Read the model definition and answer for the solid it produces. Units are mm, in the model's axes. A direction names the side the tool comes from. Coordinates: 2 decimals unless noted, no trailing zeros. Write each loop counter-clockwise with the first axis right and the second up, starting at its lowest first coordinate (ties: lowest second). Pieces come first, ordered by that corner, then holes.
(1) Which of the six approach directions +Z, -Z, +X, -X, +Y, -Y give full straight-line access (tool end or side, diameter ignored) to faces 1 (the flat face through (-7, 7, -49)), 2 (the flat face through (-13, 7, -49)), 3 (the flat face through (16, -15, 37.5)), 4 (the flat face through (0, -18, 20)), 5 (the flat face through (-6, 15, -27.5))?
(2) The mould has two halves that part along Z. Classify faces 6 (the cylindrical face through (-35.994, 14.93, -57.236)), 7 (the flat face through (11, 10, 57)), 8 (the flat face through (-16, -16, -3)): +Z half, -Z half, draft (parallel to the pull), parting line (faces both ways), or undercut.
(3) Section A-A on x = 20 is taken. Write down the section's boundary in (y, z), then the cut area to 4 significant figures.
(4) Section C-C on z = -57.5 is taken. Write down the section's boundary in (x, y).
(5) Find the intervals of material crossed by probe 1 along Z at (x, y) = (20, 17); probe 2 along Z at (x, y) = (35, 13); probe 3 along Y at (x, z) = (20, 11), in increasing order.
(6) Section B-B on y = 15 is taken. Write down the section's boundary in (x, z), then the cut area to 3 significant figures.
(7) Section D-D on x = -30 is taken. Write down the section's boundary in (y, z).
(8) Given pin 1 (3 mm diameter, centred on y = 7, z = 57, fed in from +X); pin 2 (3 mm diameter, centred on y = -40, z = -15, fed in from +X); pin 3 (14 mm diameter, centred on x = 20, z = -57.5, fed in from -Y), each flat-ended and moving along its own axis, determine where each tip first touches the part or whether it passes through.
Solid Edge part; units mm, degrees
sketch "Sketch1" plane through (0, 0, 0) normal (0, 0, 1) x (1, 0, 0)
  line L0 (-50, 0) -> (0, 0)
  line L1 (0, 0) -> (0, -36.6)
  arc A0 (0, -36.6) -> (40, -36.6) centre (20, -36.6) ccw
  line L2 (-50, 0) -> (6.5476, -51.3997)
extrude "Protrusion1" add sketch "Sketch1" along normal mid plane 6 material side at (-25, -0.05, 0)
sketch "Sketch2" plane through (0, 0, 0) normal (0, 0, 1) x (1, 0, 0)
  line L0 (40, 20) -> (-50, 20)
  line L1 (-50, 20) -> (-50, 0)
  line L2 (-50, 0) -> (0, 0)
  line L3 (0, 0) -> (0, -36.6)
  arc A0 (0, -36.6) -> (40, -36.6) centre (20, -36.6) ccw
  line L4 (40, -36.6) -> (40, 20)
  circle A1 centre (20, -36.6) radius 10
extrude "ExtrudedProtrusion_2" add sketch "Sketch2" along normal mid plane 75
sketch "Sketch3" plane through (0, 0, 0) normal (0, 0, 1) x (1, 0, 0)
  line L0 (-50, 10) -> (40, 10)
  line L1 (40, 10) -> (40, 20)
  line L2 (40, 20) -> (-50, 20)
  line L3 (-50, 20) -> (-50, 10)
extrude "ExtrudedCutout_4" cut sketch "Sketch3" along normal mid plane 55
sketch "Sketch4" plane through (-5, -18.3, 37.5) normal (0, 0, 1) x (0, 1, 0)
  line L0 (38.3, 45) -> (28.3, 45)
  line L1 (28.3, 45) -> (28.3, -45)
  line L2 (28.3, -45) -> (38.3, -45)
  line L3 (38.3, -45) -> (38.3, 45)
extrude "ExtrudedProtrusion_5" add sketch "Sketch4" along normal blind 40
sketch "Sketch5" plane through (40, 20, -37.5) normal (0, 0, -1) x (0, -1, 0)
  line L0 (10, 0) -> (0, 0)
  line L1 (0, 0) -> (0, 90)
  line L2 (0, 90) -> (10, 90)
  line L3 (10, 90) -> (10, 0)
extrude "ExtrudedProtrusion_6" add sketch "Sketch5" along normal blind 40
sketch "Sketch6" plane through (-5, 10, 57.5) normal (0, -1, 0) x (1, 0, 0)
  circle A0 centre (25, 0) radius 6
  circle A1 centre (-25, 0) radius 6
  circle A2 centre (25, -115) radius 6
  circle A3 centre (-25, -115) radius 6
extrude "ExtrudedCutout_5" cut sketch "Sketch6" against normal blind 100
sketch "Sketch7" plane through (-13, 10, 0) normal (-1, 0, 0) x (0, 0, -1)
  line L0 (-77.5, 0) -> (-37.5, 10)
  line L1 (-37.5, 10) -> (-37.5, 0)
  line L2 (-37.5, 0) -> (-77.5, 0)
  line L3 (37.5, 10) -> (77.5, 0)
  line L4 (77.5, 0) -> (37.5, 0)
  line L5 (37.5, 0) -> (37.5, 10)
extrude "ExtrudedProtrusion_7" add sketch "Sketch7" against normal blind 6
Response:
1. face 1: -Z, +X, -Y
1. face 2: -Z, -X, -Y
1. face 3: +Z, +X, -Y
1. face 4: +Z, -X, -Y
1. face 5: +X, -X, +Y
2. face 6: undercut
2. face 7: draft
2. face 8: -Z half
3. outline: (-56.6, -37.5) - (-46.6, -37.5) - (-46.6, 37.5) - (-56.6, 37.5) - close; (-26.6, -37.5) - (10, -37.5) - (10, -51.5) - (20, -51.5) - (20, -27.5) - (10, -27.5) - (10, 27.5) - (20, 27.5) - (20, 51.5) - (10, 51.5) - (10, 37.5) - (-26.6, 37.5) - close; (10, -77.5) - (20, -77.5) - (20, -63.5) - (10, -63.5) - close; (10, 63.5) - (20, 63.5) - (20, 77.5) - (10, 77.5) - close
3. area: 4,255 mm2
4. outline: (-50, 10) - (-36, 10) - (-36, 20) - (-50, 20) - close; (-24, 10) - (-13, 10) - (-13, 5) - (-7, 5) - (-7, 10) - (14, 10) - (14, 20) - (-24, 20) - close; (26, 10) - (40, 10) - (40, 20) - (26, 20) - close
5. probe 1: z = -77.5 to -63.5, -51.5 to -27.5, 27.5 to 51.5, 63.5 to 77.5
5. probe 2: z = -77.5 to -27.5, 27.5 to 77.5
5. probe 3: y = -56.6 to -46.6, -26.6 to 10
6. outline: (-50, -77.5) - (40, -77.5) - (40, -27.5) - (-50, -27.5) - close; (-50, 27.5) - (40, 27.5) - (40, 77.5) - (-50, 77.5) - close; hole circle Ø12 at (-30, -57.5); hole circle Ø12 at (-30, 57.5); hole circle Ø12 at (20, -57.5); hole circle Ø12 at (20, 57.5)
6. area: 8,550 mm2
7. outline: (-18.18, -3) - (0, -3) - (0, -37.5) - (10, -37.5) - (10, -51.5) - (20, -51.5) - (20, -27.5) - (10, -27.5) - (10, 27.5) - (20, 27.5) - (20, 51.5) - (10, 51.5) - (10, 37.5) - (0, 37.5) - (0, 3) - (-18.18, 3) - close; (10, -77.5) - (20, -77.5) - (20, -63.5) - (10, -63.5) - close; (10, 63.5) - (20, 63.5) - (20, 77.5) - (10, 77.5) - close
8. pin 1: stops at x = -7
8. pin 2: stops at x = 39.91
8. pin 3: stops at y = 10
